Here's how the part is built. I have some questions about the finished solid (model axes, mm). Coordinates: 2 decimals unless noted, no trailing zeros. Loops run counter-clockwise (first coordinate to the right, second up) from the corner with the lowest first, then second, coordinate; pieces in that order, holes last. Notation, with made-up numbers: (-33.75, 29) -> (-4.75, 29) arc R27 ccw to (-4.75, 67) -> close; hole circle Ø10 at (86.25, -19.5). An arc over 180 degrees is marked (long way). Answer as a JSON object with one key per item and string values. Group by question number.
Q1. Thinking about a two-plate mould opening in Z: for faces 1 (the flat face through (42, 19, 0)), 2 (the flat face through (36, 19, -3.175)), 3 (the flat face through (0, 19, -23)), which applies, released by +Z, released by -Z, zero draft, split by the parting line, or undercut?
Q2. I need wall thicknesses on line 1 (X direction, y = 12.5, z = -23) (3 decimals); line 2 (X direction, y = 3, z = -15.5) (3 decimals); line 3 (Z direction, x = 37.5, y = 26.5) (3 decimals). Which ranges of each line are inside material? Lowest first, please.
Q3. I want a section at C-C on y = 18. Write out the boundary of the cut face in (x, z) (3 decimals).
Q4. I want a section at D-D on z = -14. Write out the boundary of the cut face in (x, y) (3 decimals).
Q5. I want a section at A-A on x = 61. Write out the boundary of the cut face in (y, z) (3 decimals).
Q6. I want a section at B-B on y = 14. Write out the boundary of the cut face in (x, z) (3 decimals).
Q7. I'm going to push flat-ended pins straight in: pin 1 (6 mm diameter, centred on x = 71, y = 28.5, fed in from -Z); pin 2 (5 mm diameter, centred on y = 13.5, z = -38.5, fed in from +X); pin 3 (11.5 mm diameter, centred on x = 41.5, y = 16, fed in from -Z). Where does each tip first touch, or does it pass through?
```python
from build123d import *

# Parameters (mm, degrees)
BOSS_EXTRUDE1_DEPTH  = 38.1
CUT_EXTRUDE1_DEPTH   = 103.587389576
M5_CLEARANCE_HOLE1_D = 5.5


with BuildPart() as part:
    # Sketch1 → Boss-Extrude1 (new body)
    with BuildSketch(Plane(origin=(0, 0, 0), x_dir=(1, 0, 0), z_dir=(0, 1, 0))):
        Polygon((0, 0), (0, 47.625), (82.48891971, 0), align=None)
    extrude(amount=BOSS_EXTRUDE1_DEPTH)

    # Sketch2 → Cut-Extrude1 (cut, through all)
    with BuildSketch(Plane(origin=(0, 38.1, 0), x_dir=(1, 0, 0), z_dir=(0, 1, 0))):
        Polygon((3.175, 3.175), (70.639658396, 3.175), (3.175, 42.125738686), align=None)
    extrude(amount=-CUT_EXTRUDE1_DEPTH, mode=Mode.SUBTRACT)

    # M5 Clearance Hole1 (through all)
    with Locations(Plane(origin=(20.622229928, 0, -35.71875), x_dir=(-0.8660254037844417, 0, -0.4999999999999947), z_dir=(0.4999999999999947, 0, -0.8660254037844417))):
        with Locations((17.4625, 12.7), (-65.0875, 12.7), (-65.0875, 25.4), (17.4625, 25.4)):
            Hole(M5_CLEARANCE_HOLE1_D / 2)


solid = part.part
```
Result set:
{
 "1": {"face 1": "released by +Z", "face 2": "undercut", "face 3": "zero draft"},
 "2": {"line 1": "x = 0 to 3.175, 36.302 to 42.652", "line 2": "x = 0 to 3.175, 49.292 to 55.642", "line 3": "z = -25.974 to -22.308, -3.175 to 0"},
 "3": {"outline": "(0, -47.625) -> (82.489, 0) -> (0, 0) -> close; hole (3.175, -42.126) -> (70.64, -3.175) -> (3.175, -3.175) -> close"},
 "4": {"outline": "(0, 0) -> (3.175, 0) -> (3.175, 38.1) -> (0, 38.1) -> close; (51.89, 0) -> (58.24, 0) -> (58.24, 38.1) -> (51.89, 38.1) -> close"},
 "5": {"outline": "(0, -12.407) -> (38.1, -12.407) -> (38.1, -8.74) -> (0, -8.74) -> close; (0, -3.175) -> (38.1, -3.175) -> (38.1, 0) -> (0, 0) -> close"},
 "6": {"outline": "(0, -47.625) -> (3.401, -45.662) -> (0, -39.772) -> close; (0, -30.078) -> (3.175, -35.578) -> (3.175, -3.175) -> (70.64, -3.175) -> (6.01, -40.489) -> (7.598, -43.238) -> (74.891, -4.387) -> (72.358, 0) -> (0, 0) -> close; (77.955, 0) -> (79.088, -1.963) -> (82.489, 0) -> close"},
 "7": {"pin 1": "stops at z = -8.37", "pin 2": "stops at x = 20.14", "pin 3": "stops at z = -26.98"}
}
